Could you check a few things on this model? Use its own coordinates, in mm. Coordinates: 2 decimals unless noted, no trailing zeros. Write each loop counter-clockwise with the first axis right and the second up, starting at its lowest first coordinate (ties: lowest second). Pieces come first, ordered by that corner, then holes.
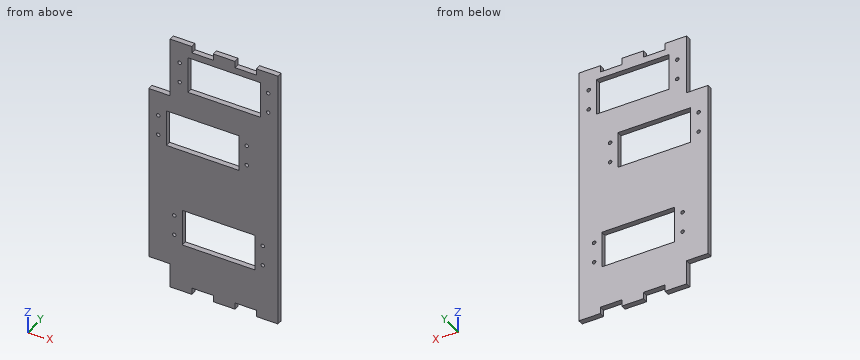
```python
from build123d import *

# Parameters (mm, degrees)
SKETCH1_W           = 40.8
SKETCH1_H           = 20.6
BOSS_EXTRUDE4_DEPTH = 3
SKETCH2_R           = 1
CUT_EXTRUDE1_DEPTH  = 4


with BuildPart() as part:
    # Sketch1 → Boss-Extrude4 (new body)
    with BuildSketch(Plane(origin=(0, 0, 0), x_dir=(1, 0, 0), z_dir=(0, 1, 0))):
        Polygon((30.25, -70), (30.25, 70), (30.25, 73.75), (18.15, 73.75), (18.15, 70), (6.05, 70), (6.05, 73.75), (-6.05, 73.75), (-6.05, 70), (-18.15, 70), (-18.15, 73.75), (-30.25, 73.75), (-30.25, 70), (-30.25, 60), (-42.25, 60), (-42.25, -40), (-30.25, -40), (-30.25, -70), (-30.25, -73.75), (-18.15, -73.75), (-18.15, -70), (-6.05, -70), (-6.05, -73.75), (6.05, -73.75), (6.05, -70), (18.15, -70), (18.15, -73.75), (30.25, -73.75), align=None)
        with Locations((0, -56)):
            Rectangle(SKETCH1_W, SKETCH1_H, mode=Mode.SUBTRACT)
        with Locations((-12, -20)):
            Rectangle(SKETCH1_W, SKETCH1_H, mode=Mode.SUBTRACT)
        with Locations((-3, 36)):
            Rectangle(SKETCH1_W, SKETCH1_H, mode=Mode.SUBTRACT)
    extrude(amount=BOSS_EXTRUDE4_DEPTH)

    # Sketch2 → Cut-Extrude1 (cut, through all)
    with BuildSketch(Plane(origin=(0, 3, 0), x_dir=(1, 0, 0), z_dir=(0, 1, 0))):
        with Locations((-25, -50.1)):
            Circle(SKETCH2_R)
        with Locations((-25, -61.6)):
            Circle(SKETCH2_R)
        with Locations((-37, -25.9)):
            Circle(SKETCH2_R)
        with Locations((-28, 30.4)):
            Circle(SKETCH2_R)
        with Locations((-28, 41.9)):
            Circle(SKETCH2_R)
        with Locations((21.7, 41.9)):
            Circle(SKETCH2_R)
        with Locations((21.7, 30.4)):
            Circle(SKETCH2_R)
        with Locations((12.7, -14.4)):
            Circle(SKETCH2_R)
        with Locations((12.7, -25.9)):
            Circle(SKETCH2_R)
        with Locations((24.7, -50.1)):
            Circle(SKETCH2_R)
        with Locations((24.7, -61.6)):
            Circle(SKETCH2_R)
        with Locations((-37, -14.4)):
            Circle(SKETCH2_R)
    extrude(amount=-CUT_EXTRUDE1_DEPTH, mode=Mode.SUBTRACT)


solid = part.part
```
1. Please list where these lines run through material, in increasing order: line 1 along Z through (x, y) = (-28, 2.25); line 2 along Z through (x, y) = (21.7, 1.3); line 3 along Z through (x, y) = (-21.5, 1.65).
Verdict:
line 1: z = -73.75 to -42.9, -40.9 to -31.4, -29.4 to 9.7, 30.3 to 73.75
line 2: z = -73.75 to -42.9, -40.9 to -31.4, -29.4 to 73.75
line 3: z = -73.75 to -46.3, -25.7 to 9.7, 30.3 to 73.75
2. I want a section at C-C on x = 4.5. Please give me the cut outline in (y, z), plus the area to 3 significant figures.
Verdict:
outline: (0, -73.75) - (3, -73.75) - (3, -46.3) - (0, -46.3) - close; (0, -25.7) - (3, -25.7) - (3, 9.7) - (0, 9.7) - close; (0, 30.3) - (3, 30.3) - (3, 45.7) - (0, 45.7) - close; (0, 66.3) - (3, 66.3) - (3, 73.75) - (0, 73.75) - close
area: 257 mm2
3. I want a section at B-B on y = 0.65. Give the number of separate pieces and of enclosed holes in the cut face, plus the area to 3 significant figures.
Verdict:
separate pieces: 1
enclosed holes: 15
area: 7,380 mm2
4. I want a section at A-A on x = -12. Please give me the cut outline in (y, z), plus the area to 3 significant figures.
Verdict:
outline: (0, -70) - (3, -70) - (3, -46.3) - (0, -46.3) - close; (0, -25.7) - (3, -25.7) - (3, 9.7) - (0, 9.7) - close; (0, 30.3) - (3, 30.3) - (3, 45.7) - (0, 45.7) - close; (0, 66.3) - (3, 66.3) - (3, 70) - (0, 70) - close
area: 235 mm2
5. For pin 1 (1.6 mm diameter, centred on x = -25, z = 50.1, fed in from -Y); pin 2 (0.9 mm diameter, centred on x = -36.5, y = 1.5, fed in from +Z); pin 3 (0.9 mm diameter, centred on x = -10, y = 1.5, fed in from -Z); pin 4 (0.9 mm diameter, centred on y = 1, z = -71.5, fed in from -X), each with a flat end and sliding along its axis, tell me the tip position at first contact or that it passes through.
Verdict:
pin 1: passes through
pin 2: stops at z = 40
pin 3: stops at z = -70
pin 4: stops at x = -30.25
